from build123d import *
from build123d.topology import SkipClean

# Parameters (mm, degrees)
SKETCH1_R           = 15.07617
BOSS_EXTRUDE1_DEPTH = 118.4446395
SKETCH2_R           = 9.3853
SKETCH2_R_2         = 4.5847
BOSS_EXTRUDE2_DEPTH = 4.7498
CUT_EXTRUDE1_DEPTH  = 26
SKETCH4_R           = 2.25
CUT_EXTRUDE2_DEPTH  = 2.6
CUT_EXTRUDE3_START  = -10
SKETCH5_R           = 15.07617
SKETCH5_R_2         = 7
CUT_EXTRUDE3_DEPTH  = 10


with BuildPart() as part:
    # Sketch1 → Boss-Extrude1 (new body)
    with BuildSketch(Plane(origin=(0, 0, 0), x_dir=(0, 0, -1), z_dir=(1, 0, 0))):
        with Locations(Location((0, 0, 0), (0, 0, 180))):
            Circle(SKETCH1_R)
    extrude(amount=BOSS_EXTRUDE1_DEPTH)

    # Sketch2 → Boss-Extrude2 (add)
    with BuildSketch(Plane.ZY):
        with Locations(Location((0, 0, 0), (0, 0, 180))):
            Circle(SKETCH2_R)
        Circle(SKETCH2_R_2, mode=Mode.SUBTRACT)
    extrude(amount=BOSS_EXTRUDE2_DEPTH)

    # Sketch3 → Cut-Extrude1 (cut)
    with BuildSketch(Plane(origin=(118.4446395, 0, 0), x_dir=(0, 0, -1), z_dir=(1, 0, 0))):
        with BuildLine():
            Line((-1.870828693, 1.25), (1.870828693, 1.25))
            ThreePointArc((1.870828693, 1.25), (0, -2.25), (-1.870828693, 1.25))
        make_face()
    extrude(amount=-CUT_EXTRUDE1_DEPTH, mode=Mode.SUBTRACT)

    # Sketch4 → Cut-Extrude2 (cut)
    with SkipClean():  # the faces are left unmerged after this step: merging them gives an invalid solid
        with BuildSketch(Plane(origin=(118.4446395, 0, 0), x_dir=(0, 0, -1), z_dir=(1, 0, 0))):
            Circle(SKETCH4_R)
        extrude(amount=-CUT_EXTRUDE2_DEPTH, mode=Mode.SUBTRACT)

    # Sketch5 → Cut-Extrude3 (cut)
    with SkipClean():  # the faces are left unmerged after this step: merging them gives an invalid solid
        with BuildSketch(Plane(origin=(118.4446395, 0, 0), x_dir=(0, 0, -1), z_dir=(1, 0, 0)).offset(CUT_EXTRUDE3_START)):
            with Locations(Location((0, 0, 0), (0, 0, 180))):
                Circle(SKETCH5_R)
            Circle(SKETCH5_R_2, mode=Mode.SUBTRACT)
        extrude(amount=CUT_EXTRUDE3_DEPTH, mode=Mode.SUBTRACT)


solid = part.part
Verification items for the finished model (mm, model axes). A direction names the side the tool comes from. Round coordinates to 2 decimals unless told otherwise and drop trailing zeros. Order: outer loops, then holes, each group sorted by start corner. A loop starts at its lowest first (then second) coordinate and runs counter-clockwise, first axis right, second up.
1. Section check A-A on z = 0. Record the cut outline in (x, y).
Final values:
outline: (-4.75, -9.39) - (0, -9.39) - (0, -15.08) - (108.44, -15.08) - (108.44, -7) - (118.44, -7) - (118.44, -2.25) - (92.44, -2.25) - (92.44, 1.25) - (115.84, 1.25) - (115.84, 2.25) - (118.44, 2.25) - (118.44, 7) - (108.44, 7) - (108.44, 15.08) - (0, 15.08) - (0, 9.39) - (-4.75, 9.39) - (-4.75, 4.58) - (0, 4.58) - (0, -4.58) - (-4.75, -4.58) - close
2. Section check C-C on x = 96. Record the cut outline in (y, z), then the cut area to 3 significant figures.
Final values:
outline: circle Ø30.15 at (0, 0); hole (1.25, -1.87) - (1.25, 1.87) arc R2.25 ccw (long way) to start
area: 701 mm2
3. Release check for a two-part mould opening along Z. For faces 4 (the flat face through (104, 1.25, 0)), 5 (the flat face through (108.445, 3.1, 6.5)), 6 (the cylindrical face through (-2.34, -2.82, -8.95)) record: +Z half, -Z half, draft (parallel to the pull), parting line (faces both ways), or undercut.
Final values:
face 4: undercut
face 5: draft
face 6: parting line
4. Section check D-D on x = 80. Record the cut outline in (y, z).
Final values:
outline: circle Ø30.15 at (0, 0)
5. Go/stop test with flat-tipped pins: P1, Ø1, axis at y = 10, z = 11.5, coming from the -X side; P2, Ø4, axis at x = 23, y = 9, coming from the -Z side; P3, Ø0.8, axis at y = 1.5, z = -0.5, coming from the +X side. Record where each tip stops, or that it passes through.
Final values:
P1: stops at x = 0
P2: stops at z = -13.35
P3: stops at x = 115.84
6. Access from +Z, -Z, +X, -X, +Y, -Y to the whole of each face (thin tool, end or side, straight path). Record for faces 1 (the flat face through (0, 10, 0)), 2 (the flat face through (118.445, -2, -2)), 3 (the cylindrical face through (113.375, -2.681, -6.466)).
Final values:
face 1: -X
face 2: +Z, -Z, +X, +Y, -Y
face 3: +X
7. Section check B-B on y = 0. Record the cut outline in (x, z).
Final values:
outline: (-4.75, -9.39) - (0, -9.39) - (0, -15.08) - (108.44, -15.08) - (108.44, -7) - (118.44, -7) - (118.44, -2.25) - (92.44, -2.25) - (92.44, 2.25) - (118.44, 2.25) - (118.44, 7) - (108.44, 7) - (108.44, 15.08) - (0, 15.08) - (0, 9.39) - (-4.75, 9.39) - (-4.75, 4.58) - (0, 4.58) - (0, -4.58) - (-4.75, -4.58) - close
8. Thickness scan on L1, parallel to Y at x = 100.75, z = 0; L2, parallel to Y at x = -3.7, z = 0; L3, parallel to X at y = -8, z = 6.5. Record the ranges inside material, lowest first.
Final values:
L1: y = -15.08 to -2.25, 1.25 to 15.08
L2: y = -9.39 to -4.58, 4.58 to 9.39
L3: x = 0 to 108.44
